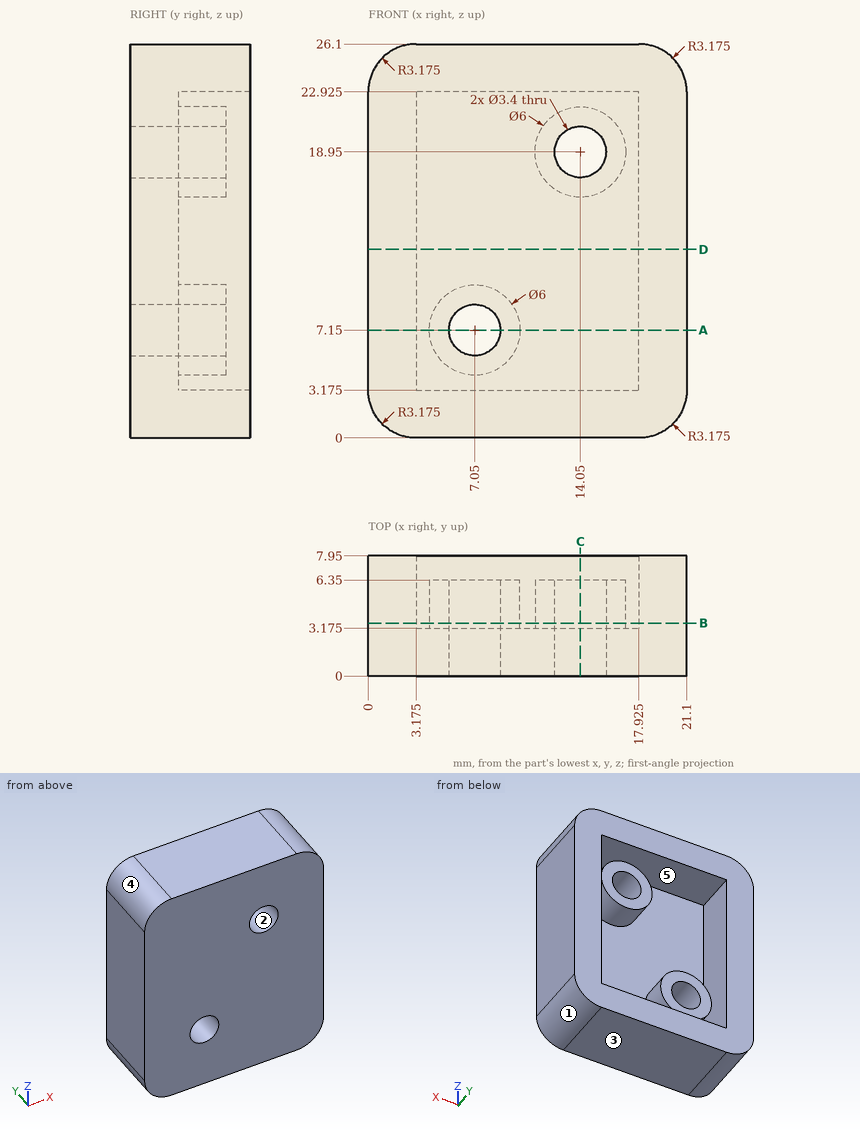
Answer from the drawing. Dimensions are ordinates in mm from the lowest x, y and z of the part. A direction names the side the tool comes from. Coordinates: 2 decimals unless noted, no trailing zeros. Loops run counter-clockwise (first coordinate to the right, second up) from the corner with the lowest first, then second, coordinate; pieces in that order, holes last. Notation, with made-up numbers: (-21.75, -21.5) -> (24.25, -21.5) arc R20 ccw to (24.25, -10.5) -> close; hole circle Ø4 at (-26.5, 58). An arc over 180 degrees is marked (long way). Answer in a Markdown table with one row per item.
Item 1: This flat-tipped pin is pushed along its axis until it touches: P1, Ø1.8, axis at x = 8.5, z = 6, coming from the +Y side. Where does it stop, or does it pass through?
Returned:
| item | result |
|---|---|
| P1 | stops at y = 6.35 |
Item 2: A cutting plane is placed at C-C on x = 14.05. Determine the outline of the cut face in (y, z) (3 decimals).
Returned:
| item | result |
|---|---|
| outline | (0, 0) -> (7.95, 0) -> (7.95, 3.175) -> (3.175, 3.175) -> (3.175, 15.95) -> (6.35, 15.95) -> (6.35, 17.25) -> (0, 17.25) -> close; (0, 20.65) -> (6.35, 20.65) -> (6.35, 21.95) -> (3.175, 21.95) -> (3.175, 22.925) -> (7.95, 22.925) -> (7.95, 26.1) -> (0, 26.1) -> close |
Item 3: A cutting plane is placed at D-D on z = 12.5. Determine the outline of the cut face in (x, y) (3 decimals), plus the area to 3 significant figures.
Returned:
| item | result |
|---|---|
| outline | (0, 0) -> (21.1, 0) -> (21.1, 7.95) -> (17.925, 7.95) -> (17.925, 3.175) -> (3.175, 3.175) -> (3.175, 7.95) -> (0, 7.95) -> close |
| area | 97.3 mm^2 |
Item 4: For a pull along X with two mould halves and no side action, classify the marked faces 1, 2 and 3 as released by +X, released by -X, zero draft, split by the parting line, or undercut.
Returned:
| item | result |
|---|---|
| face 1 | released by +X |
| face 2 | undercut |
| face 3 | zero draft |
Item 5: Straight lines are drawn through the part: line 1 along Z through (x, y) = (7.05, 4.75) (3 decimals); line 2 along Z through (x, y) = (5.5, 6.75) (3 decimals); line 3 along Z through (x, y) = (7.05, 3). For each, find the intervals that lie inside material, in ascending order. Write a range as [from, to].
Returned:
| item | result |
|---|---|
| line 1 | z = [0, 3.175], [4.15, 5.45], [8.85, 10.15], [22.925, 26.1] |
| line 2 | z = [0, 3.175], [22.925, 26.1] |
| line 3 | z = [0, 5.45], [8.85, 26.1] |
Item 6: A cutting plane is placed at A-A on z = 7.15. Determine the outline of the cut face in (x, y) (3 decimals).
Returned:
| item | result |
|---|---|
| outline | (0, 0) -> (5.35, 0) -> (5.35, 6.35) -> (4.05, 6.35) -> (4.05, 3.175) -> (3.175, 3.175) -> (3.175, 7.95) -> (0, 7.95) -> close; (8.75, 0) -> (21.1, 0) -> (21.1, 7.95) -> (17.925, 7.95) -> (17.925, 3.175) -> (10.05, 3.175) -> (10.05, 6.35) -> (8.75, 6.35) -> close |
Item 7: A cutting plane is placed at B-B on y = 3.5. Determine the outline of the cut face in (x, z) (3 decimals), plus the area to 3 significant figures.
Returned:
| item | result |
|---|---|
| outline | (0, 3.175) arc R3.175 ccw to (3.175, 0) -> (17.925, 0) arc R3.175 ccw to (21.1, 3.175) -> (21.1, 22.925) arc R3.175 ccw to (17.925, 26.1) -> (3.175, 26.1) arc R3.175 ccw to (0, 22.925) -> close; circle Ø6 at (7.05, 7.15); circle Ø6 at (14.05, 18.95); hole (3.175, 3.175) -> (17.925, 3.175) -> (17.925, 22.925) -> (3.175, 22.925) -> close; hole circle Ø3.4 at (7.05, 7.15); hole circle Ø3.4 at (14.05, 18.95) |
| area | 289 mm^2 |
Item 8: For the marked faces 4 and 5, determine the directions among +Z, -Z, +X, -X, +Y, -Y from which every point of the face is accessible in a straight line to the end or side of a thin tool.
Returned:
| item | result |
|---|---|
| face 4 | +Z, -X, +Y, -Y |
| face 5 | +Y |
